```python
from build123d import *

# Parameters (mm, degrees)
FILLET1_R           = 0.2
FILLET2_R           = 1
SKETCH2_R           = 3
BOSS_EXTRUDE1_DEPTH = 20
CUT_EXTRUDE1_DEPTH  = 2.3


with BuildPart() as part:
    # Sketch1 → Revolve1 (revolve)
    with BuildSketch(Plane.XY):
        with BuildLine():
            Line((0, 0), (5.1, 0))
            Line((5.1, 0), (5.1, 1))
            ThreePointArc((5.1, 1), (4.1560785, 2.346833852), (2.75, 3.2))
            Line((2.75, 3.2), (0, 3.2))
            Line((0, 3.2), (0, 0))
        make_face()
    revolve(axis=Axis((0, 55, 0), (0, -1, 0)))

    # Fillet1
    fillet1_edges = [part.edges().sort_by_distance(p)[0] for p in [
        (-5.1, 0, 0),
    ]]
    fillet(fillet1_edges, radius=FILLET1_R)

    # Fillet2
    fillet2_edges = [part.edges().sort_by_distance(p)[0] for p in [
        (-5.1, 1, 0),
    ]]
    fillet(fillet2_edges, radius=FILLET2_R)

    # Sketch2 → Boss-Extrude1 (add)
    with BuildSketch(Plane.XZ):
        Circle(SKETCH2_R)
    extrude(amount=BOSS_EXTRUDE1_DEPTH)

    # Sketch6 → Revolve2 (revolve)
    with BuildSketch(Plane.XY):
        Polygon((0, 0), (0, 3.2), (2.75, 3.2), (4.9, 0), align=None)
    revolve(axis=Axis((0, 55, 0), (0, -1, 0)))

    # Sketch7 → Cut-Extrude1 (cut)
    with BuildSketch(Plane(origin=(0, 3.2, 0), x_dir=(1, 0, 0), z_dir=(0, 1, 0))):
        Polygon((1.154700538, -2), (2.309401077, 0), (1.154700538, 2), (-1.154700538, 2), (-2.309401077, 0), (-1.154700538, -2), align=None)
    extrude(amount=-CUT_EXTRUDE1_DEPTH, mode=Mode.SUBTRACT)

    # Sketch8 → Cut-Revolve1 (revolve, cut)
    with BuildSketch(Plane.XY):
        with BuildLine():
            Line((0, 0.9), (0, 0.5))
            Line((0, 0.5), (0.25, 0.5))
            ThreePointArc((0.25, 0.5), (1.298943849, 0.600925763), (2.309401077, 0.9))
            Line((2.309401077, 0.9), (0, 0.9))
        make_face()
    revolve(axis=Axis((0, 55, 0), (0, -1, 0)), mode=Mode.SUBTRACT)

    # Sketch9 → Cut-Revolve2 (revolve, cut)
    with BuildSketch(Plane.XY):
        with BuildLine():
            ThreePointArc((0, 2.814442262), (1.388448304, 2.911300775), (2.75, 3.2))
            Line((2.75, 3.2), (0, 3.2))
            Line((0, 3.2), (0, 2.814442262))
        make_face()
    revolve(axis=Axis((0, 55, 0), (0, -1, 0)), mode=Mode.SUBTRACT)


solid = part.part
```
The model under review builds one solid part; all positions refer to its coordinate system, in mm. A direction names the side the tool comes from. Round coordinates to 2 decimals unless told otherwise and drop trailing zeros. Write each loop counter-clockwise with the first axis right and the second up, starting at its lowest first coordinate (ties: lowest second). Pieces come first, ordered by that corner, then holes. Notation, with made-up numbers: M 88,58 L 121,58 A22 ccw 121,84 Z; hole C -26.5,-20.5 d2. An arc over 180 degrees is marked long. Use CSV: the item, a comma, the result in double quotes. Start each with the question number.
(1) For line 1 along Y through (x, z) = (-2, 0); line 2 along Y through (x, z) = (-0.5, -3.75); line 3 along X through (y, z) = (-7, 1), list the stretches that pass through material, from the lowest coordinate up.
(2) Clearance check with flat-ended pins moving along their axes: P1, Ø1.1, axis at x = 0.5, y = 2.5, coming from the -Z side; P2, Ø4, axis at x = 2, y = -3.5, coming from the -Z side; P3, Ø1.5, axis at y = -1, z = 3.5, coming from the -X side. State where each tip first meets the part, or that it passes through.
(3) We need section A-A, the plane y = -7.5. State the section outline as (x, z) points.
(4) Tool access review of faces 1 (the face through (-3, -10, 0)), 2 (the face through (1.74, 2.01, -0.99)), 3 (the face through (0, -20, 0)): name each direction out of +Z, -Z, +X, -X, +Y, -Y from which nothing blocks a thin tool from reaching the whole face with its end or side.
Findings:
1,line 1,"-20 to 0.79"
1,line 2,"0 to 2.66"
1,line 3,"-2.83 to 2.83"
2,P1,"z = -4.5"
2,P2,"z = -3"
2,P3,"x = -1.2"
3,outline,"C 0,0 d6"
4,face 1,"-Y"
4,face 2,"+Y"
4,face 3,"+Z, -Z, +X, -X, -Y"
